Study the drawing (mm; zero at the part's minimum x, y, z) and answer. Give positions to 0.01 mm unless a question says otherwise; leave off trailing zeros. Order: outer loops, then holes, each group sorted by start corner. A loop starts at its lowest first (then second) coordinate and runs counter-clockwise, first axis right, second up.
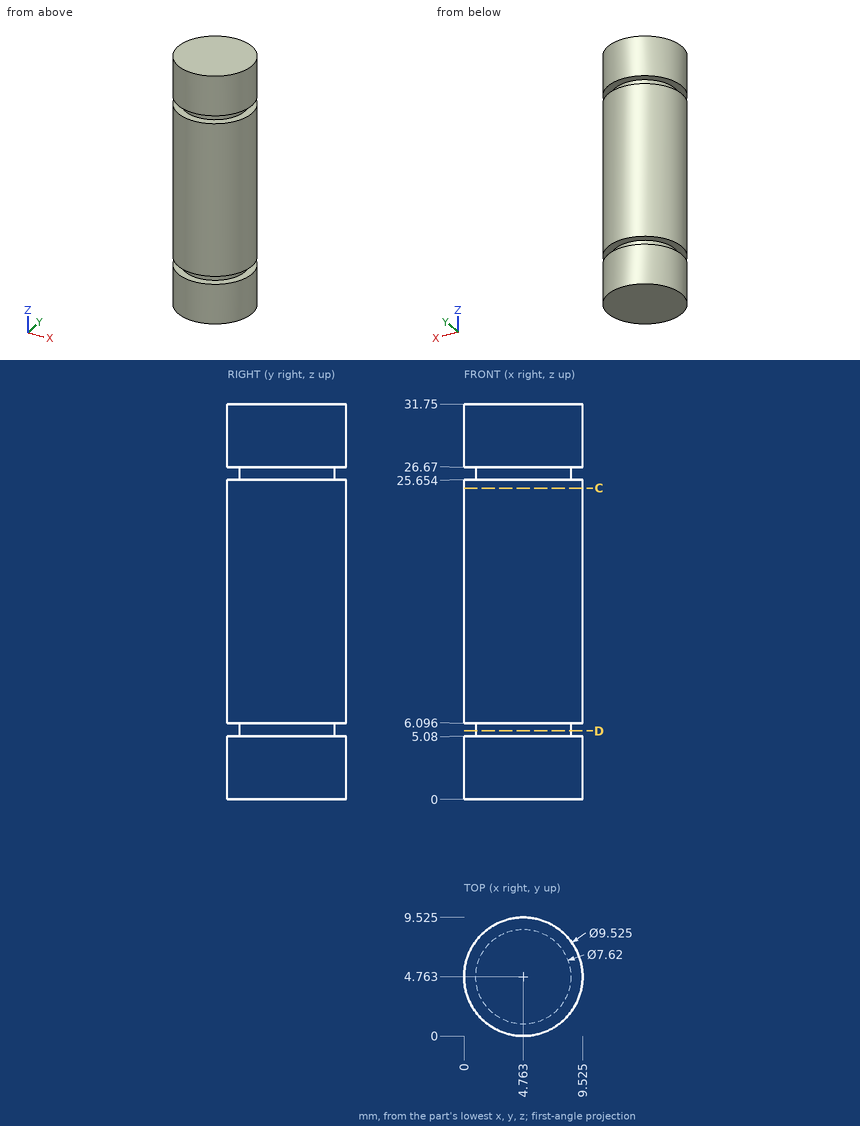
1) Find section D-D (z = 5.5). Write down the section's boundary in (x, y).
Geometry says:
outline: circle Ø7.62 at (4.76, 4.76)
2) Straight lines are drawn through the part: probe 1 along X at (y, z) = (4.5, 11.5); probe 2 along X at (y, z) = (3.75, 26.5) (1 decimal); probe 3 along Y at (x, z) = (4, 18). For each, find the intervals that lie inside material, in ascending order.
Geometry says:
probe 1: x = 0.01 to 9.52
probe 2: x = 1.1 to 8.4
probe 3: y = 0.06 to 9.46
3) Given P1, Ø3, axis at x = 6.5, z = 23, coming from the -Y side; P2, Ø4, axis at y = 2.5, z = 17.5, coming from the +X side, each flat-ended and moving along its own axis, determine where each tip first touches the part or whether it passes through.
Geometry says:
P1: stops at y = 0.01
P2: stops at x = 9.52
4) Find section C-C (z = 25). Write down the section's boundary in (x, y) (1 decimal).
Geometry says:
outline: circle Ø9.5 at (4.8, 4.8)
